```python
from build123d import *

# Parameters (mm, degrees)
EXTRUDE_1_DEPTH        = 15
FILLET_1_R             = 3
EXTRUDE_2_DEPTH        = 5
EXTRUDE_2_DEPTH_BACK   = 35
HOLE_WIZARD_M4_1_D     = 3
HOLE_WIZARD_M4_2_D     = 8
HOLE_WIZARD_M4_2_DEPTH = 13
HOLE_WIZARD_M4_2_TIP   = 2.403442476


with BuildPart() as part:
    # 스케치1 → 보스-돌출1 (new body, symmetric)
    with BuildSketch(Plane.XY):
        Polygon((0, 0), (-20, 0), (-43, 14), (-43, 30), (0, 30), align=None)
    extrude(amount=EXTRUDE_1_DEPTH, both=True)

    # 필렛1
    fillet_1_edges = [part.edges().sort_by_distance(p)[0] for p in [
        (-43, 30, 0),
        (0, 30, 0),
    ]]
    fillet(fillet_1_edges, radius=FILLET_1_R)

    # 스케치2 → 보스-돌출2 (add, two sides)
    with BuildSketch(Plane.XY.offset(15)) as extrude_2_sk:
        Polygon((-43, 27), (0, 27), (0, 3), (-24.928571429, 3), (-43, 14), align=None)
    extrude(amount=EXTRUDE_2_DEPTH)
    extrude(extrude_2_sk.sketch, amount=-EXTRUDE_2_DEPTH_BACK)

    # M4 여유 구멍1 (through all)
    with Locations(Plane.XY.offset(20)):
        with Locations((-5, 18)):
            Hole(HOLE_WIZARD_M4_1_D / 2)

    # M4 여유 구멍2
    with Locations(Plane(origin=(0, 0, 0), x_dir=(0, 0, -1), z_dir=(1, 0, 0))):
        with Locations((0, 14)):
            Hole(HOLE_WIZARD_M4_2_D / 2, depth=HOLE_WIZARD_M4_2_DEPTH)
            with Locations((0, 0, -(HOLE_WIZARD_M4_2_DEPTH + HOLE_WIZARD_M4_2_TIP / 2))):  # 118° drill point
                Cone(0, HOLE_WIZARD_M4_2_D / 2, HOLE_WIZARD_M4_2_TIP, mode=Mode.SUBTRACT)


solid = part.part
```
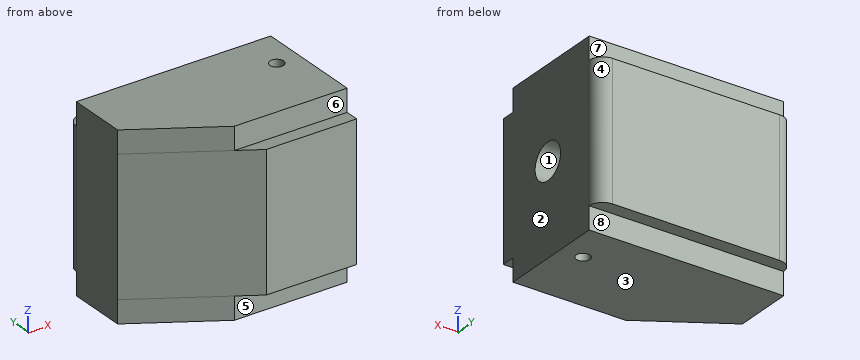
The model under review builds one solid part; all positions refer to its coordinate system, in mm. Face numbers are marked on the shaded views. A direction names the side the tool comes from. Coordinates: 2 decimals unless noted, no trailing zeros. Order: outer loops, then holes, each group sorted by start corner. A loop starts at its lowest first (then second) coordinate and runs counter-clockwise, first axis right, second up. Notation, with made-up numbers: (-19.5, 4) -> (31.5, 4) arc R28 cw to (31.5, 25) -> close; hole circle Ø9 at (85.25, 32.5). An arc over 180 degrees is marked (long way). Answer in a Markdown table with one row per item. Add a question column.
Item 1: Machinability: for the marked faces 4, 5, 6, 7 and 8, which of the approach directions +Z, -Z, +X, -X, +Y, -Y give a long, thin tool a straight path to every point of the face, cutting with its end or side? Answer none if there is none.
Item 2: Clearance check with flat-ended pins moving along their axes: pin 1 (1 mm diameter, centred on y = 10.5, z = 8, fed in from -X); pin 2 (2.5 mm diameter, centred on x = -13, y = 29, fed in from +Z); pin 3 (5.5 mm diameter, centred on x = -14.5, z = -18, fed in from +Y). State where each tip first meets the part, or that it passes through.
Item 3: We need section C-C on x = -33. Write out the cut boundary in (y, z).
Item 4: We need section D-D on y = 6.75. Write out the cut boundary in (x, z), plus the area to 3 significant figures.
Item 5: To check wall thickness, follow probe 1 along X at (y, z) = (18, -4); probe 2 along Z at (x, y) = (-3.5, 14); probe 3 along Y at (x, z) = (-5, 9.5). State the ranges of each line that lie inside material, in increasing order.
Item 6: We need section A-A on x = -8. Write out the cut boundary in (y, z).
Item 7: We need section B-B on z = 9. Write out the cut boundary in (x, y).
Item 8: Mouldability with a two-part tool opening along Z and no side actions: class the marked faces 1, 2 and 3 as +Z half, -Z half, draft (parallel to the pull), parting line (faces both ways), or undercut.
Final values:
| question | item | result |
|---|---|---|
| 1 | face 4 | +Z, -Z, +X, +Y |
| 1 | face 5 | -Z, +X, -X, -Y |
| 1 | face 6 | +Z, +X, -X, -Y |
| 1 | face 7 | +Z, +X, -X, +Y |
| 1 | face 8 | -Z, +X, -X, +Y |
| 2 | pin 1 | stops at x = -38.07 |
| 2 | pin 2 | stops at z = 15 |
| 2 | pin 3 | stops at y = 27 |
| 3 | outline | (7.91, -20) -> (27, -20) -> (27, -15) -> (30, -15) -> (30, 15) -> (27, 15) -> (27, 20) -> (7.91, 20) -> close |
| 4 | outline | (-31.09, -20) -> (0, -20) -> (0, 20) -> (-31.09, 20) -> close |
| 4 | area | 1,240 mm2 |
| 5 | probe 1 | x = -43 to -6.5, -3.5 to 0 |
| 5 | probe 2 | z = -20 to -4, 4 to 20 |
| 5 | probe 3 | y = 0 to 16.5, 19.5 to 30 |
| 6 | outline | (0, -15) -> (3, -15) -> (3, -20) -> (27, -20) -> (27, -15) -> (30, -15) -> (30, 15) -> (27, 15) -> (27, 20) -> (3, 20) -> (3, 15) -> (0, 15) -> close; hole circle Ø8 at (14, 0) |
| 7 | outline | (-43, 14) -> (-20, 0) -> (0, 0) -> (0, 27) arc R3 ccw to (-3, 30) -> (-40, 30) arc R3 ccw to (-43, 27) -> close; hole circle Ø3 at (-5, 18) |
| 8 | face 1 | undercut |
| 8 | face 2 | draft |
| 8 | face 3 | -Z half |
